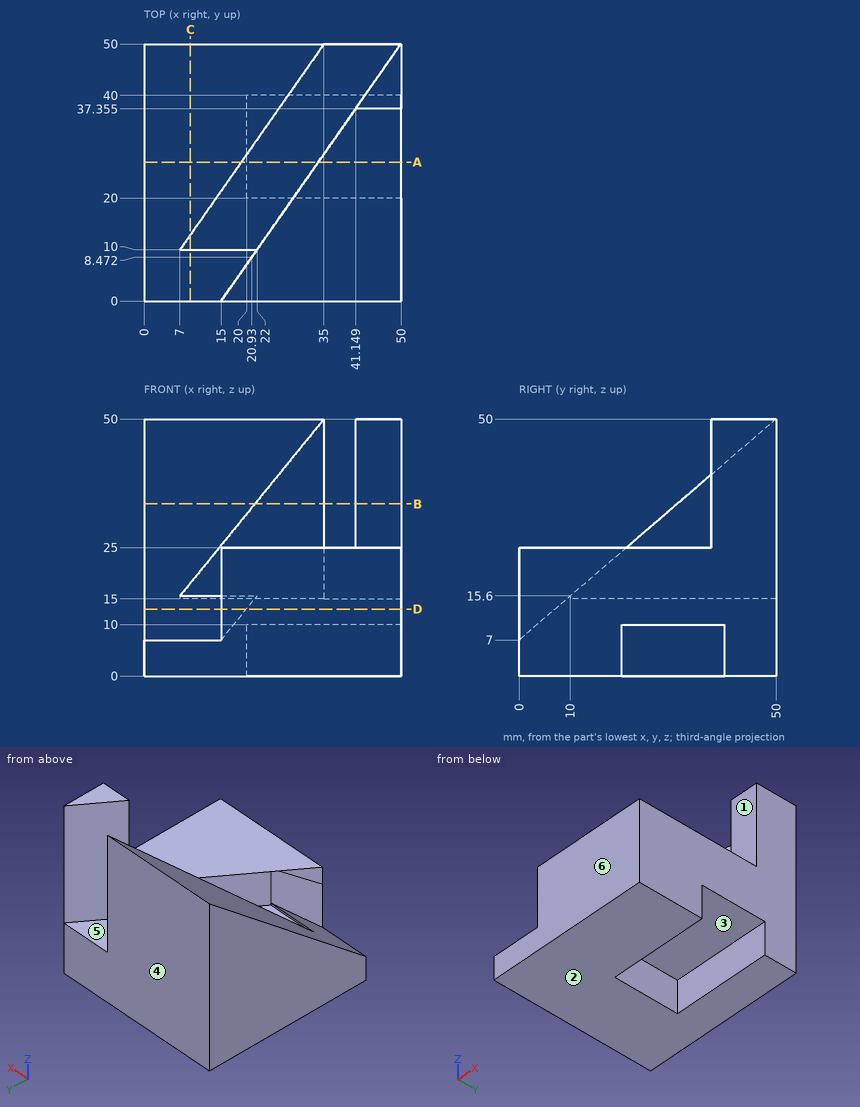
Study the drawing (mm; zero at the part's minimum x, y, z) and answer. A direction names the side the tool comes from. Round coordinates to 2 decimals unless told otherwise and drop trailing zeros. Loops run counter-clockwise (first coordinate to the right, second up) from the corner with the lowest first, then second, coordinate; pieces in that order, holes last. Notation, with made-up numbers: (74.5, -13) -> (115.5, -13) arc R8 ccw to (115.5, -7) -> close; hole circle Ø2 at (11, 58). An arc over 180 degrees is marked (long way). Write each question's results on one line, items separated by ' | '. Start each with the question number.
1. A tool of negligible diameter and unlimited length cuts with its end or side. For the marked faces 1, 2 and 3, from which of +Z, -Z, +X, -X, +Y, -Y can it reach the whole face along a straight path? Write none if from no direction.
2. For a pull along Y with two mould halves and no side action, classify the marked faces 4, 5 and 6 as +Y half, -Y half, draft (parallel to the pull), parting line (faces both ways), or undercut.
3. Section B-B (z = 33.5) is taken. Determine the outline of the cut face in (x, y) (1 decimal).
4. Section D-D (z = 13) is taken. Determine the outline of the cut face in (x, y), plus the area to 3 significant figures.
5. Find the intervals of material crossed by probe 1 along Z at (x, y) = (40, 31); probe 2 along Y at (x, z) = (46, 7.5); probe 3 along X at (y, z) = (20.5, 16.5), in increasing order. Write a range as from..to.
6. Given pin 1 Ø1 at (x, y) = (15, 14.5) entering from +Z; pin 2 Ø16 at (x, y) = (28.5, 34) entering from -Z; pin 3 Ø5 at (x, y) = (38.5, 33.5) entering from -Z; pin 4 Ø9.5 at (x, z) = (47, 36) entering from -Y (1 decimal), each flat-ended and moving along its own axis, determine where each tip first touches the part or whether it passes through.
7. Section A-A (y = 27) is taken. Determine the outline of the cut face in (x, z).
8. Section C-C (x = 9) is taken. Determine the outline of the cut face in (y, z), plus the area to 3 significant figures.
Evaluation:
1) face 1: +Z, +X, -Y | face 2: -Z, +X, -X, +Y, -Y | face 3: -Z, +X
2) face 4: +Y half | face 5: undercut | face 6: -Y half
3) outline: (0, 30.8) -> (21.6, 30.8) -> (35, 50) -> (0, 50) -> close; (41.1, 37.4) -> (50, 37.4) -> (50, 50) -> close
4) outline: (0, 6.98) -> (19.88, 6.98) -> (15, 0) -> (50, 0) -> (50, 50) -> (0, 50) -> close | area: 2,380 mm2
5) probe 1: z = 10..25 | probe 2: y = 0..20, 40..50 | probe 3: x = 0..14.35, 29.35..50
6) pin 1: stops at z = 15 | pin 2: stops at z = 0 | pin 3: stops at z = 10 | pin 4: stops at y = 37.4
7) outline: (0, 0) -> (20, 0) -> (20, 10) -> (50, 10) -> (50, 25) -> (33.9, 25) -> (33.9, 15) -> (18.9, 15) -> (18.9, 30.22) -> (0, 30.22) -> close
8) outline: (0, 0) -> (50, 0) -> (50, 50) -> (12.86, 18.06) -> (12.86, 15) -> (10, 15) -> (10, 15.6) -> (0, 7) -> close | area: 1,420 mm2
